Here's the drawing with two shaded views (mm, measured from the low corner). I have some questions. A direction names the side the tool comes from. Round coordinates to 2 decimals unless told otherwise and drop trailing zeros. Loops run counter-clockwise (first coordinate to the right, second up) from the corner with the lowest first, then second, coordinate; pieces in that order, holes last. Notation, with made-up numbers: (47, 73.5) -> (96, 73.5) arc R14 ccw to (96, 77.5) -> close; hole circle Ø2 at (13.5, -8). An arc over 180 degrees is marked (long way). Write item = value, one per line.
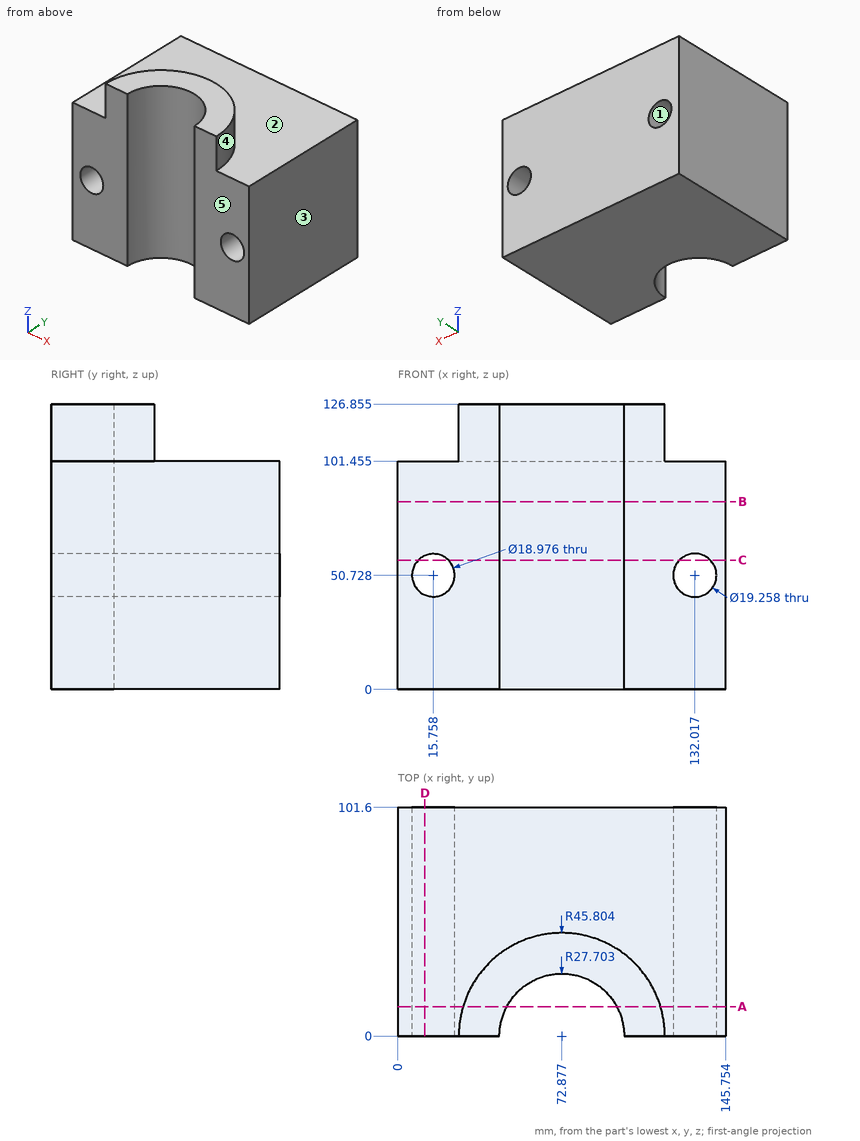
1. For the marked faces 4 and 5, which set-ups out of +Z, -Z, +X, -X, +Y, -Y let a thin tool reach every point of the face, with its end or its side?
Entries:
face_4 = +Z, +Y
face_5 = +Z, -Z, +X, -X, -Y
2. I need wall thicknesses on line 1 (X direction, y = 6.5, z = 102); line 2 (Y direction, x = 71.5, z = 27.5); line 3 (Z direction, x = 124, y = 78.5) (1 decimal). Which ranges of each line are inside material? Lowest first, please. Write a range as [from, to].
Entries:
line_1 = [27.54, 45.95], [99.81, 118.22]
line_2 = [27.67, 101.6]
line_3 = [0, 45.4], [56.1, 101.5]
3. Suppose I cut it at C-C, the plane z = 57.5. List the corners of the cut face in (x, y) for me (1 decimal).
Entries:
outline = (0, 0) -> (9.1, 0) -> (9.1, 101.6) -> (0, 101.6) -> close; (22.4, 0) -> (45.2, 0) arc R27.7 cw to (100.6, 0) -> (125.2, 0) -> (125.2, 101.6) -> (22.4, 101.6) -> close; (138.9, 0) -> (145.8, 0) -> (145.8, 101.6) -> (138.9, 101.6) -> close
4. We'd pull the mould along X, two halves only. Please class the marked faces 1, 2 and 3: released by +X, released by -X, zero draft, split by the parting line, or undercut.
Entries:
face_1 = undercut
face_2 = zero draft
face_3 = released by +X
5. Suppose I cut it at B-B, the plane z = 83.5. List the corners of the cut face in (x, y) for me (1 decimal), and give its area (3 significant figures).
Entries:
outline = (0, 0) -> (45.2, 0) arc R27.7 cw to (100.6, 0) -> (145.8, 0) -> (145.8, 101.6) -> (0, 101.6) -> close
area = 13,600 mm²
6. Suppose I cut it at D-D, the plane x = 12. List the corners of the cut face in (y, z) for me (1 decimal), and give its area (3 significant figures).
Entries:
outline = (0, 0) -> (101.6, 0) -> (101.6, 42) -> (0, 42) -> close; (0, 59.4) -> (101.6, 59.4) -> (101.6, 101.5) -> (0, 101.5) -> close
area = 8,540 mm²
7. I'm going to push flat-ended pins straight in: pin 1 (10 mm diameter, centred on y = 13, z = 82.5, fed in from -X); pin 2 (10 mm diameter, centred on x = 28.5, y = 57.5, fed in from +Z) (1 decimal). Where does each tip first touch, or does it pass through?
Entries:
pin_1 = 0
pin_2 = 101.5
8. Suppose I cut it at A-A, the plane y = 13. List the corners of the cut face in (x, z) for me (1 decimal), and give its area (3 significant figures).
Entries:
outline = (0, 0) -> (48.4, 0) -> (48.4, 126.9) -> (29, 126.9) -> (29, 101.5) -> (0, 101.5) -> close; (97.3, 0) -> (145.8, 0) -> (145.8, 101.5) -> (116.8, 101.5) -> (116.8, 126.9) -> (97.3, 126.9) -> close; hole circle Ø19 at (15.8, 50.7); hole circle Ø19.3 at (132, 50.7)
area = 10,200 mm²
